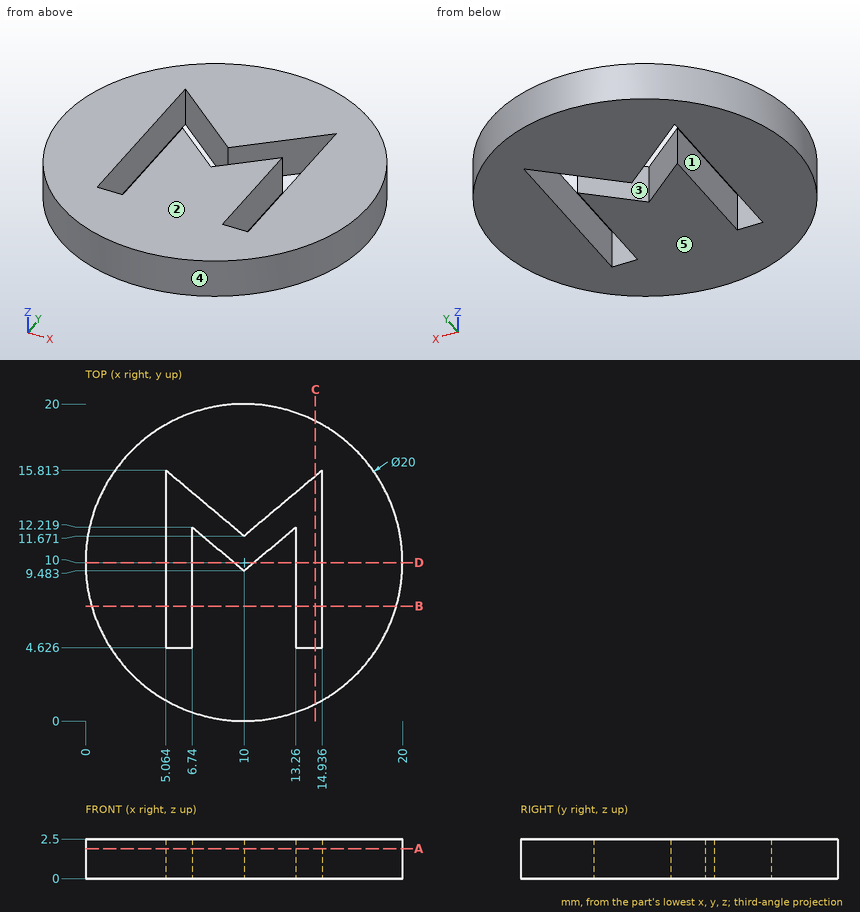
Here's the drawing with two shaded views (mm, measured from the low corner). I have some questions. A direction names the side the tool comes from. Round coordinates to 2 decimals unless told otherwise and drop trailing zeros. Order: outer loops, then holes, each group sorted by start corner. A loop starts at its lowest first (then second) coordinate and runs counter-clockwise, first axis right, second up. Notation, with made-up numbers: (55, 1.25) -> (68, 1.25) arc R14 cw to (68, 28.25) -> close; hole circle Ø5 at (49, -10). An arc over 180 degrees is marked (long way). Use a Markdown table: item, result. Add a question column.
(1) Suppose I cut it at A-A, the plane z = 1.9. Please give me the cut outline in (x, y) (1 decimal), and give its area (3 significant figures).
(2) I need wall thicknesses on line 1 along X through (y, z) = (15.25, 2.2) (1 decimal); line 2 along X through (y, z) = (12.5, 0.9) (1 decimal); line 3 along X through (y, z) = (11.25, 2.35) (1 decimal). Which ranges of each line are inside material? Lowest first, please.
(3) For the marked faces 1 and 2, which set-ups out of +Z, -Z, +X, -X, +Y, -Y let a thin tool reach every point of the face, with its end or its side?
(4) Suppose I cut it at C-C, the plane x = 14.5. Please give me the cut outline in (y, z), and give its area (3 significant figures).
(5) Suppose I cut it at B-B, the plane y = 7.25. Please give me the cut outline in (x, z) (1 decimal).
(6) For pin 1 Ø1.2 at (y, z) = (9, 1.5) entering from +X; pin 2 Ø0.8 at (x, z) = (6, 1) entering from +Y; pin 3 Ø1 at (x, z) = (2.5, 1) entering from -Y, each with a flat end and sliding along its axis, tell me the tip position at first contact or that it passes through.
(7) Suppose I cut it at D-D, the plane y = 10. Please give me the cut outline in (x, z) (1 decimal).
(8) If we mould it in two halves opening along X, with no side actions, what happens to the marked faces 3, 4 and 5? For each: released by +X, released by -X, zero draft, split by the parting line, or undercut.
Verdict:
| question | item | result |
|---|---|---|
| 1 | outline | circle Ø20 at (10, 10); hole (5.1, 4.6) -> (6.7, 4.6) -> (6.7, 12.2) -> (10, 9.5) -> (13.3, 12.2) -> (13.3, 4.6) -> (14.9, 4.6) -> (14.9, 15.8) -> (10, 11.7) -> (5.1, 15.8) -> close |
| 1 | area | 265 mm2 |
| 2 | line 1 | 1.5 to 5.1, 5.7 to 14.3, 14.9 to 18.5 |
| 2 | line 2 | 0.3 to 5.1, 9 to 11, 14.9 to 19.7 |
| 2 | line 3 | 0.1 to 5.1, 6.7 to 7.9, 12.1 to 13.3, 14.9 to 19.9 |
| 3 | face 1 | +Z, -Z |
| 3 | face 2 | +Z, +X, -X, +Y, -Y |
| 4 | outline | (1.07, 0) -> (4.63, 0) -> (4.63, 2.5) -> (1.07, 2.5) -> close; (15.45, 0) -> (18.93, 0) -> (18.93, 2.5) -> (15.45, 2.5) -> close |
| 4 | area | 17.6 mm2 |
| 5 | outline | (0.4, 0) -> (5.1, 0) -> (5.1, 2.5) -> (0.4, 2.5) -> close; (6.7, 0) -> (13.3, 0) -> (13.3, 2.5) -> (6.7, 2.5) -> close; (14.9, 0) -> (19.6, 0) -> (19.6, 2.5) -> (14.9, 2.5) -> close |
| 6 | pin 1 | x = 19.99 |
| 6 | pin 2 | y = 19.33 |
| 6 | pin 3 | y = 2.86 |
| 7 | outline | (0, 0) -> (5.1, 0) -> (5.1, 2.5) -> (0, 2.5) -> close; (6.7, 0) -> (9.4, 0) -> (9.4, 2.5) -> (6.7, 2.5) -> close; (10.6, 0) -> (13.3, 0) -> (13.3, 2.5) -> (10.6, 2.5) -> close; (14.9, 0) -> (20, 0) -> (20, 2.5) -> (14.9, 2.5) -> close |
| 8 | face 3 | undercut |
| 8 | face 4 | split by the parting line |
| 8 | face 5 | zero draft |
